Design review of the part built by this model. Coordinates are the model's own, in mm. A direction names the side the tool comes from. Coordinates: 2 decimals unless noted, no trailing zeros. Loops run counter-clockwise (first coordinate to the right, second up) from the corner with the lowest first, then second, coordinate; pieces in that order, holes last. Notation, with made-up numbers: (52, 60.25) - (83, 60.25) arc R37 cw to (83, 96.25) - close; hole circle Ø10 at (-29, -35). An arc over 180 degrees is marked (long way). Use one line per item in the form item = value. Start each with the question number.
(1) Add section B-B (z = 2.7). State the section outline as (x, y) points.
(2) Tool access review of faces 1 (the face through (376, 118, 0)), 2 (the face through (367, 120.988, 3)): name each direction out of +Z, -Z, +X, -X, +Y, -Y from which nothing blocks a thin tool from reaching the whole face with its end or side.
(3) Clearance check with flat-ended pins moving along their axes: pin 1 Ø2 at (x, z) = (366, 4.5) entering from +Y; pin 2 Ø2 at (y, z) = (119.5, 1.5) entering from +X. State where each tip first meets the part, or that it passes through.
(4) For L1, parallel to X at y = 118.25, z = 1; L2, parallel to X at y = 118.75, z = 5.05; L3, parallel to Y at x = 384.5, z = 5.65, list the stretches that pass through material, from the lowest coordinate up.
(5) The part is to be moulded in two halves that separate along Y. For faces 3 (the face through (376, 118, 5.994)), 4 (the face through (367, 114.994, 3)), 5 (the face through (361.19, 118.2, 2.96)), say which applies: pulls with the +Y half, pulls with the -Y half, needs draft (parallel to the pull), parting line crosses it, or undercut.
(6) Add section A-A (x = 368.25). State the section outline as (y, z) points, plus the area to 3 significant figures.
(7) Add section D-D (x = 386.75). State the section outline as (y, z) points, plus the area to 3 significant figures.
(8) Add section C-C (y = 120). State the section outline as (x, z) points, plus the area to 3 significant figures.
```python
from build123d import *

# Parameters (mm, degrees)
SKETCH1_W           = 5.9944
SKETCH1_H           = 5.9944
BOSS_EXTRUDE1_DEPTH = 5.9944


with BuildPart() as part:
    # Sketch1 → Boss-Extrude1 (new body)
    with BuildSketch(Plane.XY):
        with BuildLine():
            Line((384.610540851, 111.993994152), (367.537765391, 111.993994152))
            ThreePointArc((367.537765391, 111.993994152), (361.187765391, 118.343994152), (367.537765391, 124.693994152))
            Line((367.537765391, 124.693994152), (384.610540851, 124.693994152))
            ThreePointArc((384.610540851, 124.693994152), (390.960540851, 118.343994152), (384.610540851, 111.993994152))
        make_face()
        with Locations((384.610540851, 117.991248441)):
            Rectangle(SKETCH1_W, SKETCH1_H, mode=Mode.SUBTRACT)
        with Locations((367.537765391, 117.991248441)):
            Rectangle(SKETCH1_W, SKETCH1_H, mode=Mode.SUBTRACT)
    extrude(amount=BOSS_EXTRUDE1_DEPTH)


solid = part.part
```
Computed values:
q1.outline = (367.54, 111.99) - (384.61, 111.99) arc R6.35 ccw to (384.61, 124.69) - (367.54, 124.69) arc R6.35 ccw to start; hole (364.54, 114.99) - (370.53, 114.99) - (370.53, 120.99) - (364.54, 120.99) - close; hole (381.61, 114.99) - (387.61, 114.99) - (387.61, 120.99) - (381.61, 120.99) - close
q2.face_1 = -Z, +X, -X, +Y, -Y
q2.face_2 = +Z, -Z
q3.pin_1 = 124.67
q3.pin_2 = 390.96
q4.L1 = 361.19 to 364.54, 370.53 to 381.61, 387.61 to 390.96
q4.L2 = 361.2 to 364.54, 370.53 to 381.61, 387.61 to 390.95
q4.L3 = 111.99 to 114.99, 120.99 to 124.69
q5.face_3 = needs draft
q5.face_4 = undercut
q5.face_5 = parting line crosses it
q6.outline = (111.99, 0) - (114.99, 0) - (114.99, 5.99) - (111.99, 5.99) - close; (120.99, 0) - (124.69, 0) - (124.69, 5.99) - (120.99, 5.99) - close
q6.area = 40.2 mm^2
q7.outline = (112.37, 0) - (114.99, 0) - (114.99, 5.99) - (112.37, 5.99) - close; (120.99, 0) - (124.32, 0) - (124.32, 5.99) - (120.99, 5.99) - close
q7.area = 35.7 mm^2
q8.outline = (361.41, 0) - (364.54, 0) - (364.54, 5.99) - (361.41, 5.99) - close; (370.53, 0) - (381.61, 0) - (381.61, 5.99) - (370.53, 5.99) - close; (387.61, 0) - (390.74, 0) - (390.74, 5.99) - (387.61, 5.99) - close
q8.area = 104 mm^2
